Geometry check sheet. Reference: the model listing, model coordinates, mm. Round coordinates to 2 decimals unless told otherwise and drop trailing zeros. Write each loop counter-clockwise with the first axis right and the second up, starting at its lowest first coordinate (ties: lowest second). Pieces come first, ordered by that corner, then holes. Notation, with made-up numbers: M 50.25,-32 L 106.25,-32 A29 cw 106.25,2 Z; hole C 18.5,52.25 d8. An arc over 180 degrees is marked long. One line per item, written item: value. Start each with the question number.
1. Section check A-A (y = -252). Record the boundary of the cut face in (x, z), and give its area (3 significant figures).
2. Scan lines: probe 1 along Z at (x, y) = (233.5, -165.5); probe 2 along X at (y, z) = (-299, -5); probe 3 along Y at (x, z) = (377.5, -4.75). Record each from-to range of solid material in increasing order. Write a range as [from, to].
3. Section check B-B (z = -3.5). Record the boundary of the cut face in (x, y), and give its area (3 significant figures).
4. Section check C-C (x = 51). Record the boundary of the cut face in (y, z).
5. Depth check by flat-ended pin: P1, Ø3, axis at x = 433.5, z = -2, coming from the -Y side; P2, Ø5.5, axis at x = 319, z = -4.5, coming from the +Y side; P3, Ø6, axis at x = 122.5, y = -50, coming from the -Z side; P4, Ø3.5, axis at x = 330.5, z = -3, coming from the -Y side. Enter the tip coordinate at first touch or a pass-through.
from build123d import *

# Parameters (mm, degrees)
EXTRUDE_1_DEPTH = 7
SKETCH_2_R      = 3
SKETCH_2_R_2    = 0.5
EXTRUDE_2_DEPTH = 7


with BuildPart() as part:
    # 草图1 → 凸台-拉伸1 (new body)
    with BuildSketch(Plane.XY):
        Polygon((0, 0), (630, 0), (630, -400), (0, -400), (0, -18.630210668), align=None)
    extrude(amount=EXTRUDE_1_DEPTH)

    # 草图2 → 凸台-拉伸2 (add)
    with BuildSketch(Plane(origin=(0, 0, 0), x_dir=(-1, 0, 0), z_dir=(0, 0, -1))):
        Polygon((-315.471142347, -300.001109882), (-245.471142347, -300.001109882), (-245.471142347, -250.001109882), (-245.471142347, -230.001109882), (-385.471142347, -230.001109882), (-385.471142347, -300.001109882), align=None)
        with Locations((-315.572226811, -278.546162476)):
            Circle(SKETCH_2_R, mode=Mode.SUBTRACT)
        with Locations((-330.572226811, -278.546162476)):
            Circle(SKETCH_2_R_2, mode=Mode.SUBTRACT)
    extrude(amount=EXTRUDE_2_DEPTH)


solid = part.part
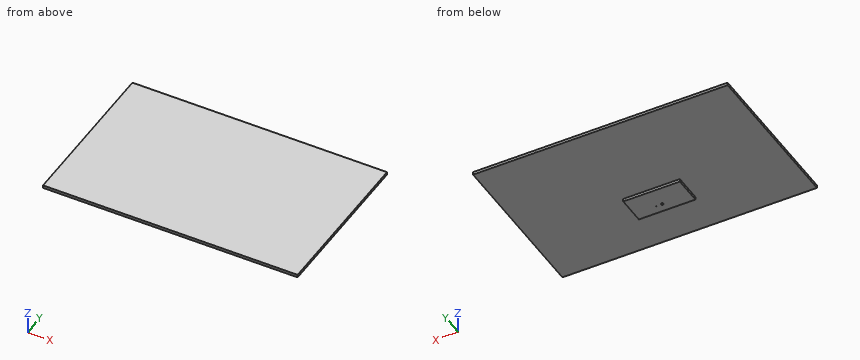
Result sheet:
1. outline: M 0,0 L 245.47,0 L 245.47,-7 L 385.47,-7 L 385.47,0 L 630,0 L 630,7 L 0,7 Z
1. area: 5,390 mm2
2. probe 1: z = [0, 7]
2. probe 2: x = [245.47, 385.47]
2. probe 3: y = [-300, -230]
3. outline: M 245.47,-300 L 385.47,-300 L 385.47,-230 L 245.47,-230 Z; hole C 315.57,-278.55 d6; hole C 330.57,-278.55 d1
3. area: 9,770 mm2
4. outline: M -400,0 L 0,0 L 0,7 L -400,7 Z
5. P1: passes through
5. P2: stops at y = -230
5. P3: stops at z = 0
5. P4: stops at y = -300
